Geometry check sheet. Reference: the model listing, model coordinates, mm. Face numbers are marked on the shaded views. A direction names the side the tool comes from. Round coordinates to 2 decimals unless told otherwise and drop trailing zeros. Write each loop counter-clockwise with the first axis right and the second up, starting at its lowest first coordinate (ties: lowest second). Pieces come first, ordered by that corner, then holes. Notation, with made-up numbers: (-27, 17.5) -> (4, 17.5) arc R28 cw to (4, 52.5) -> close; hole circle Ø5 at (-25, -12.75). An arc over 180 degrees is marked (long way). Put each result on its own line as item: value. Start each with the question number.
from build123d import *

# Parameters (mm, degrees)
F0_W      = 50.8
F0_H      = 50.8
F1_DEPTH  = 7.62
F2_T      = -1.27
F3_W      = 1.27
F3_H      = 31.657300781
F3_H_2    = 7.62
F3_H_3    = 12.7
F3_W_2    = 19.05
F3_H_4    = 1.27
F3_H_5    = 19.05
F3_W_3    = 12.7
F3_W_4    = 2.54
F3_H_6    = 2.54
F4_DEPTH  = 6.35
F5_R      = 1.27
F6_DEPTH  = 25.4
F7_R      = 1.27
F8_DEPTH  = 25.4
F9_R      = 1.27
F10_DEPTH = 25.4
F11_R     = 1.27
F12_DEPTH = 25.4


with BuildPart() as f1:
    # F0 (on Top) → F1 (new body)
    with BuildSketch(Plane.XY):
        with Locations((25.4, 25.4)):
            Rectangle(F0_W, F0_H)
    extrude(amount=-F1_DEPTH)

    # F2
    f2_openings = [f1.faces().sort_by_distance(p)[0] for p in [
        (25.4, 25.4, 0),
    ]]
    offset(amount=F2_T, openings=f2_openings)

    # F3 (on face) → F4 (join)
    with BuildSketch(Plane.XY.offset(-6.35)):
        with Locations((6.985, 17.0986503905)):
            Rectangle(F3_W, F3_H)
        Polygon((6.35, 34.197300781), (6.35, 32.927300781), (7.62, 32.927300781), (20.32, 32.927300781), (20.32, 41.817300781), (19.05, 41.817300781), (19.05, 34.197300781), align=None)
        with Locations((6.985, 45.72)):
            Rectangle(F3_W, F3_H_2)
        with Locations((29.7986493057, 43.18)):
            Rectangle(F3_W, F3_H_3)
        with Locations((40.005, 29.8451691666)):
            Rectangle(F3_W_2, F3_H_4)
        with Locations((37.4186493057, 43.18)):
            Rectangle(F3_W, F3_H_3)
        with Locations((16.496093998, 10.795)):
            Rectangle(F3_W, F3_H_5)
        with Locations((43.18, 14.0302554315)):
            Rectangle(F3_W_3, F3_H_4)
        with Locations((25.515874902, 7.62)):
            Rectangle(F3_W, F3_H_3)
        with Locations((22.1276638252, 25.3072996777)):
            Rectangle(F3_W_4, F3_H_6)
    extrude(amount=F4_DEPTH)

    # F5 (on face) → F6 (cut)
    with BuildSketch(Plane.XY.offset(-6.35)):
        with Locations((33.2517512143, 45.72)):
            Circle(F5_R)
    extrude(amount=-F6_DEPTH, mode=Mode.SUBTRACT)

    # F7 (on face) → F8 (cut)
    with BuildSketch(Plane.XY.offset(-6.35)):
        with Locations((12.051093998, 7.1008764207)):
            Circle(F7_R)
    extrude(amount=-F8_DEPTH, mode=Mode.SUBTRACT)

    # F9 (on face) → F10 (cut)
    with BuildSketch(Plane.XY.offset(-6.35)):
        with Locations((3.81, 3.81)):
            Circle(F9_R)
    extrude(amount=-F10_DEPTH, mode=Mode.SUBTRACT)

    # F11 (on face) → F12 (cut)
    with BuildSketch(Plane.XY.offset(-6.35)):
        with Locations((3.81, 10.16)):
            Circle(F11_R)
    extrude(amount=-F12_DEPTH, mode=Mode.SUBTRACT)


solid = f1.part
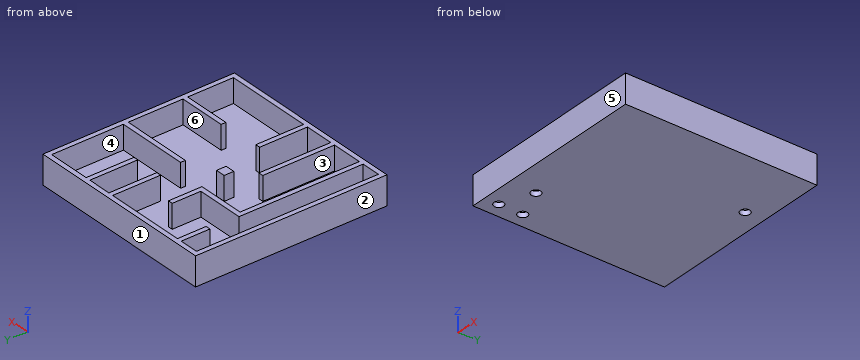
(1) Sectioned sample at B-B (x = 3.81). Record the cut outline in (y, z).
(2) Sectioned sample at D-D (x = 45.5). Record the cut outline in (y, z).
(3) Mould release check, pull along X, two halves, no side actions. Record for the marked faces 1, 2, 3 and 4: +X half, -X half, draft (parallel to the pull), parting line (faces both ways), or undercut.
(4) Material ranges on L1, parallel to X at y = 41, z = -4.75; L2, parallel to X at y = 7, z = -1.25; L3, parallel to X at y = 34.5, z = -4.5, recorded low to high. Write a range as from..to.
(5) Sectioned sample at A-A (y = 45.72). Record the cut outline in (x, z), and give its area (3 significant figures).
(6) Set-up check for the marked faces 5 and 6: record each of +Z, -Z, +X, -X, +Y, -Y from which the full face is reachable in a straight line by a thin tool's end or side.
(7) Sectioned sample at C-C (z = -3.75). State how many separate pieces and enclosed holes the cut face has, and give its area (3 significant figures).
(8) Go/stop test with flat-tipped pins: pin 1 Ø2 at (x, y) = (3.81, 3.81) entering from +Z; pin 2 Ø2 at (x, y) = (45.5, 25) entering from +Z. Record where each tip stops, or that it passes through.
Found:
1. outline: (0, -7.62) -> (2.54, -7.62) -> (2.54, -6.35) -> (1.27, -6.35) -> (1.27, 0) -> (0, 0) -> close; (5.08, -7.62) -> (8.89, -7.62) -> (8.89, -6.35) -> (5.08, -6.35) -> close; (11.43, -7.62) -> (50.8, -7.62) -> (50.8, 0) -> (49.53, 0) -> (49.53, -6.35) -> (11.43, -6.35) -> close
2. outline: (0, -7.62) -> (50.8, -7.62) -> (50.8, 0) -> (49.53, 0) -> (49.53, -6.35) -> (30.48, -6.35) -> (30.48, 0) -> (29.21, 0) -> (29.21, -6.35) -> (14.67, -6.35) -> (14.67, 0) -> (13.4, 0) -> (13.4, -6.35) -> (1.27, -6.35) -> (1.27, 0) -> (0, 0) -> close
3. face 1: draft
3. face 2: -X half
3. face 3: undercut
3. face 4: undercut
4. L1: 0..1.27, 19.05..20.32, 29.16..30.43, 36.78..38.05, 49.53..50.8
4. L2: 0..1.27, 6.35..7.62, 15.86..17.13, 24.88..26.15, 49.53..50.8
4. L3: 0..1.27, 19.05..20.32, 49.53..50.8
5. outline: (0, -7.62) -> (31.98, -7.62) -> (31.98, -6.35) -> (30.43, -6.35) -> (30.43, 0) -> (29.16, 0) -> (29.16, -6.35) -> (7.62, -6.35) -> (7.62, 0) -> (6.35, 0) -> (6.35, -6.35) -> (1.27, -6.35) -> (1.27, 0) -> (0, 0) -> close; (34.52, -7.62) -> (50.8, -7.62) -> (50.8, 0) -> (49.53, 0) -> (49.53, -6.35) -> (38.05, -6.35) -> (38.05, 0) -> (36.78, 0) -> (36.78, -6.35) -> (34.52, -6.35) -> close
5. area: 102 mm2
6. face 5: +Z, -Z, +X, -X, -Y
6. face 6: +Z
7. separate pieces: 2
7. enclosed holes: 1
7. area: 448 mm2
8. pin 1: through
8. pin 2: z = -6.35
